Can you work these out from the drawing? Everything is in mm from the part's minimum corner. Coordinates: 2 decimals unless noted, no trailing zeros. Order: outer loops, then holes, each group sorted by start corner. A loop starts at its lowest first (then second) coordinate and runs counter-clockwise, first axis right, second up. Notation, with made-up numbers: M 52,67 L 111,67 A16 ccw 111,86 Z; hole C 77.25,-3.5 d11. An arc over 180 degrees is marked long. Answer as a JSON object with one key per item and string values.
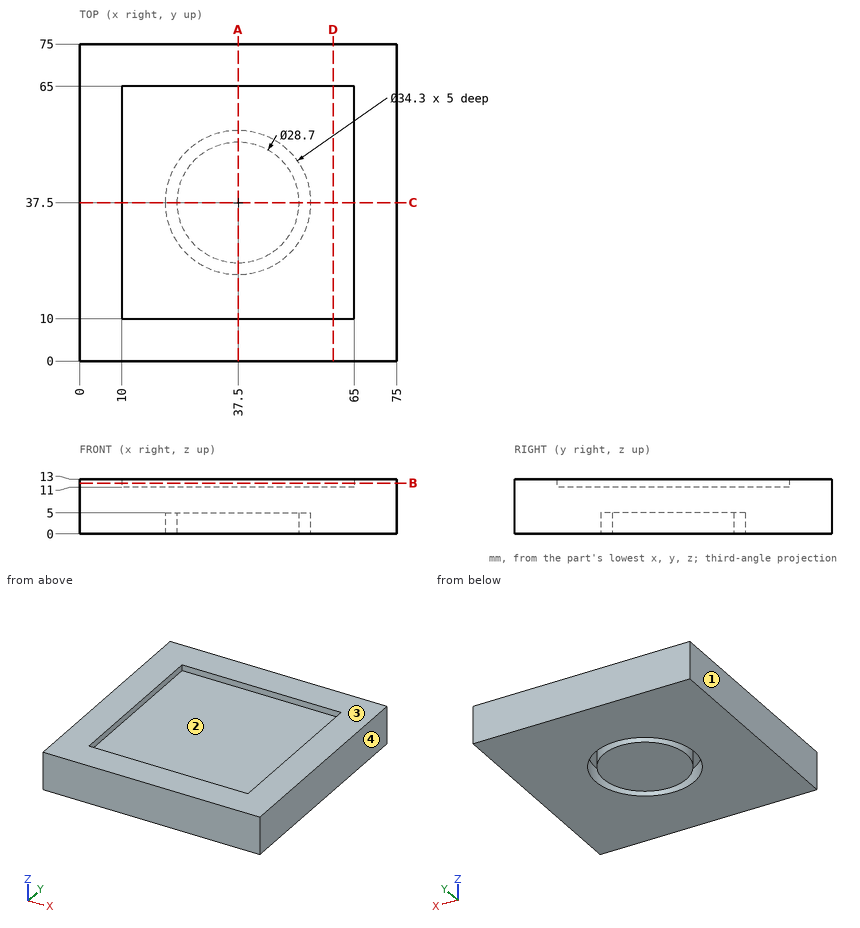
Item 1: I'm going to push a flat-ended pin straight in: pin 1 (20.5 mm diameter, centred on x = 37.5, y = 37.5, fed in from +Z). Where does the tip first touch, or does it pass through?
Answers follow:
{"pin 1": "stops at z = 11"}
Item 2: I want a section at D-D, the plane x = 60. Write out the boundary of the cut face in (y, z).
Answers follow:
{"outline": "M 0,0 L 75,0 L 75,13 L 65,13 L 65,11 L 10,11 L 10,13 L 0,13 Z"}
Item 3: Please list where these lines run through material, in increasing order: line 1 (Y direction, x = 37.5, z = 2.5); line 2 (Y direction, x = 57, z = 12.25); line 3 (Y direction, x = 47, z = 3.5).
Answers follow:
{"line 1": "y = 0 to 20.35, 23.15 to 51.85, 54.65 to 75", "line 2": "y = 0 to 10, 65 to 75", "line 3": "y = 0 to 23.22, 26.74 to 48.26, 51.78 to 75"}
Item 4: If we mould it in two halves opening along X, with no side actions, what happens to the marked faces 1, 2, 3 and 4? For each: pulls with the +X half, pulls with the -X half, needs draft (parallel to the pull), parting line crosses it, or undercut.
Answers follow:
{"face 1": "pulls with the -X half", "face 2": "undercut", "face 3": "needs draft", "face 4": "pulls with the +X half"}
Item 5: I want a section at A-A, the plane x = 37.5. Write out the boundary of the cut face in (y, z), plus the area to 3 significant figures.
Answers follow:
{"outline": "M 0,0 L 20.35,0 L 20.35,5 L 23.15,5 L 23.15,0 L 51.85,0 L 51.85,5 L 54.65,5 L 54.65,0 L 75,0 L 75,13 L 65,13 L 65,11 L 10,11 L 10,13 L 0,13 Z", "area": "837 mm^2"}
Item 6: I want a section at B-B, the plane z = 12. Write out the boundary of the cut face in (x, y), plus the area to 3 significant figures.
Answers follow:
{"outline": "M 0,0 L 75,0 L 75,75 L 0,75 Z; hole M 10,10 L 65,10 L 65,65 L 10,65 Z", "area": "2,600 mm^2"}
